```python
from build123d import *

# Parameters (mm, degrees)
SKETCH1_R           = 0.889
BOSS_EXTRUDE1_DEPTH = 6.35


with BuildPart() as part:
    # Sketch1 → Boss-Extrude1 (new body)
    with BuildSketch(Plane(origin=(0, 0, 0), x_dir=(1, 0, 0), z_dir=(0, 1, 0))):
        with BuildLine():
            Line((-32.390505008, 10.370660171), (-22.421005008, 10.370660171))
            ThreePointArc((-22.421005008, 10.370660171), (-21.298472993, 9.905692187), (-20.833505008, 8.783160171))
            Line((-20.833505008, 8.783160171), (-20.833505008, 2.918160067))
            ThreePointArc((-20.833505008, 2.918160067), (-21.298472993, 1.795628052), (-22.421005008, 1.330660067))
            Line((-22.421005008, 1.330660067), (-28.072941082, 1.330660067))
            ThreePointArc((-28.072941082, 1.330660067), (-28.680451031, 1.209818825), (-29.195473097, 0.865692083))
            Line((-29.195473097, 0.865692083), (-31.925537023, -1.864371844))
            ThreePointArc((-31.925537023, -1.864371844), (-32.440559089, -2.208498586), (-33.048069038, -2.329339829))
            Line((-33.048069038, -2.329339829), (-42.550505008, -2.329339829))
            ThreePointArc((-42.550505008, -2.329339829), (-44.795569038, -1.399403859), (-45.725505008, 0.845660171))
            Line((-45.725505008, 0.845660171), (-45.725505008, 2.750660171))
            Line((-45.725505008, 2.750660171), (-43.815505008, 2.750660171))
            Line((-43.815505008, 2.750660171), (-43.815505008, 4.050660171))
            Line((-43.815505008, 4.050660171), (-45.720505008, 4.050660171))
            Line((-45.720505008, 4.050660171), (-45.720505008, 4.850660171))
            Line((-45.720505008, 4.850660171), (-37.220505008, 4.850660171))
            Line((-37.220505008, 4.850660171), (-37.220505008, 4.050660171))
            Line((-37.220505008, 4.050660171), (-39.125505008, 4.050660171))
            Line((-39.125505008, 4.050660171), (-39.125505008, 2.750660171))
            Line((-39.125505008, 2.750660171), (-35.565505008, 2.750660171))
            Line((-35.565505008, 2.750660171), (-35.565505008, 7.195660171))
            ThreePointArc((-35.565505008, 7.195660171), (-34.635569038, 9.440724202), (-32.390505008, 10.370660171))
        make_face()
        with Locations(Location((-32.390505008, 5.850660171, 0), (0, 0, 270))):
            Circle(SKETCH1_R, mode=Mode.SUBTRACT)
        with Locations(Location((-22.865505008, 5.850660171, 0), (0, 0, 270))):
            Circle(SKETCH1_R, mode=Mode.SUBTRACT)
    extrude(amount=BOSS_EXTRUDE1_DEPTH)


solid = part.part
```
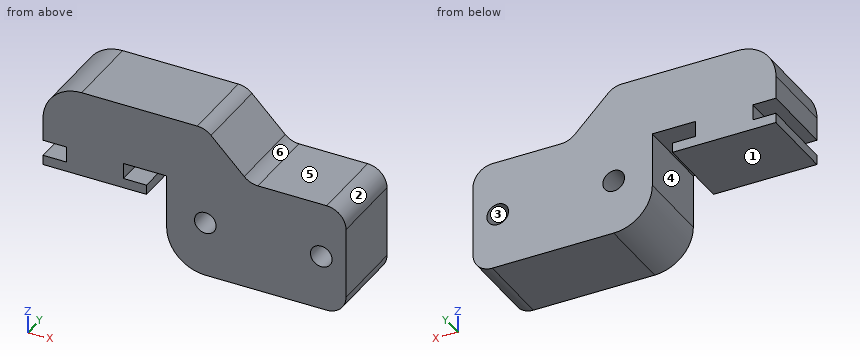
Geometry: final body of the model. Coordinates: model frame, mm. Face numbers are marked on the shaded views. A direction names the side the tool comes from. Coordinates: 2 decimals unless noted, no trailing zeros. Order: outer loops, then holes, each group sorted by start corner. A loop starts at its lowest first (then second) coordinate and runs counter-clockwise, first axis right, second up. Notation, with made-up numbers: (23.25, 89) -> (63.25, 89) arc R7 cw to (63.25, 96) -> close; hole circle Ø5 at (31.25, 83.5). An arc over 180 degrees is marked (long way). Write each question's results on one line, items separated by ' | '. Start each with the question number.
1) Cut plane D-D, the plane z = -0.25. Output: boundary loops of the cut face in (x, y), and give its area (3 significant figures).
2) Cut plane A-A, the plane z = -6. Output: boundary loops of the cut face in (x, y), and give its area (3 significant figures).
3) Cut plane B-B, the plane y = 5.25. State how many separate pieces and enclosed holes the cut face has, and give its area (3 significant figures).
4) Material intervals for line 1 along X through (y, z) = (1, -4.75); line 2 along X through (y, z) = (4.75, -4); line 3 along Z through (x, y) = (-38.5, 1.25), sorted ascending.
5) Mould query, pull axis X, two halves, no side actions, for the marked faces 3, 4, 5 and 6. Classes: released by +X, released by -X, zero draft, split by the parting line, or undercut.
6) Cut plane C-C, the plane x = -41. Output: boundary loops of the cut face in (y, z).
7) Set-up query: the marked faces 1 and 2. Return all of +Z, -Z, +X, -X, +Y, -Y with unobstructed straight access to the full face (end or side cutting, diameter ignored); none if empty.
8) First-contact query: pin 1 (1 mm diameter, centred on x = -45, y = 3.5, fed in from +Z); pin 2 (3 mm diameter, centred on y = 1, z = -1, fed in from +X); pin 3 (3.5 mm diameter, centred on y = 3, z = -5, fed in from -X). Flat tips, straight axial feed; report the tip coordinate or a pass-through.
Checks:
1) outline: (-45.67, 0) -> (-29.81, 0) -> (-29.81, 6.35) -> (-45.67, 6.35) -> close | area: 101 mm^2
2) outline: (-35.57, 0) -> (-33.27, 0) -> (-33.27, 6.35) -> (-35.57, 6.35) -> close; (-31.51, 0) -> (-23.74, 0) -> (-23.74, 6.35) -> (-31.51, 6.35) -> close; (-21.99, 0) -> (-20.83, 0) -> (-20.83, 6.35) -> (-21.99, 6.35) -> close | area: 71.3 mm^2
3) separate pieces: 1 | enclosed holes: 2 | area: 206 mm^2
4) line 1: -45.72 to -37.22, -35.57 to -20.83 | line 2: -43.82 to -39.13, -35.57 to -20.83 | line 3: -4.85 to -4.05, -2.75 to 2.33
5) face 3: undercut | face 4: undercut | face 5: zero draft | face 6: released by +X
6) outline: (0, -4.85) -> (6.35, -4.85) -> (6.35, 2.33) -> (0, 2.33) -> close
7) face 1: -Z, -X, +Y, -Y | face 2: +Z, +X, +Y, -Y
8) pin 1: z = 1.66 | pin 2: x = -20.89 | pin 3: x = -45.72
